Can you work these out from the drawing? Everything is in mm from the part's minimum corner. A direction names the side the tool comes from. Give positions to 0.01 mm unless a question says otherwise; leave off trailing zeros. One line per question, with ' | ' between items.
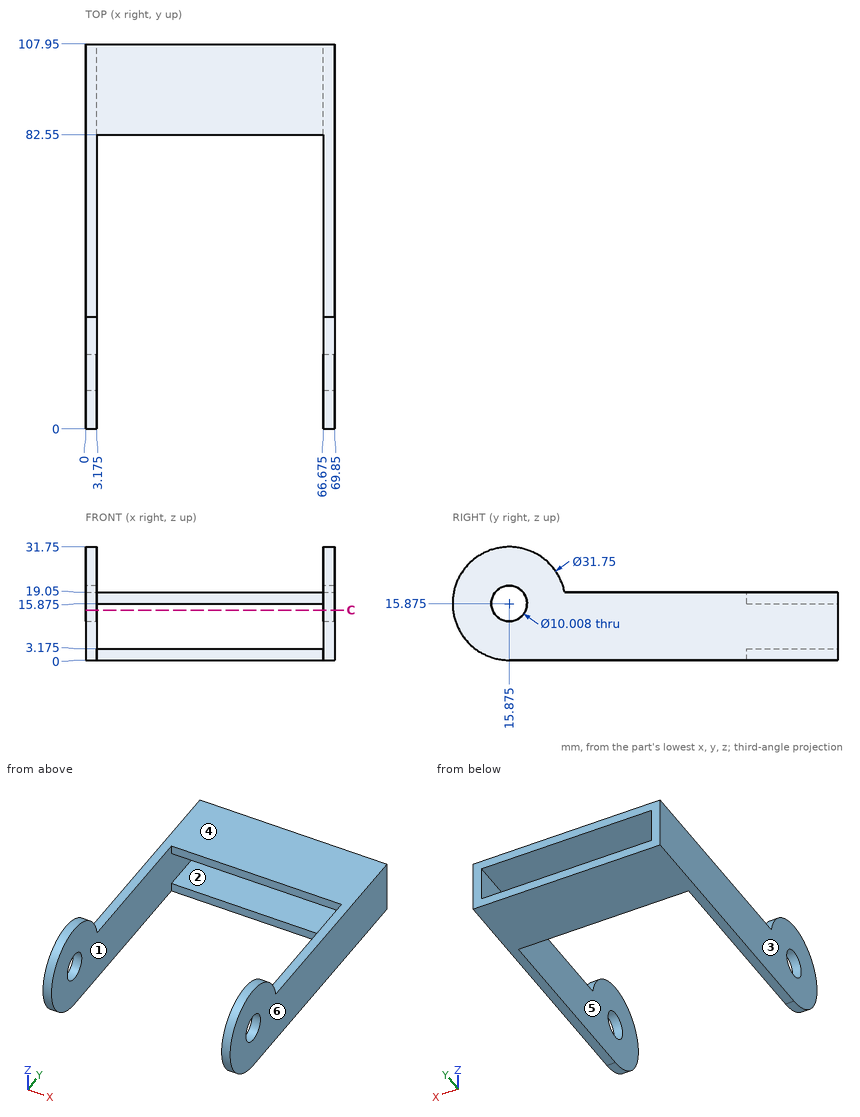
1) Thinking about a two-plate mould opening in X: for the marked faces 4, 5 and 6, which applies, +X half, -X half, draft (parallel to the pull), parting line (faces both ways), or undercut?
Model answer:
face 4: draft | face 5: undercut | face 6: +X half
2) On a 3-axis mill with a long thin cutter (end or side, diameter ignored), from which of +Z, -Z, +X, -X, +Y, -Y can I reach the whole of each face in a straight line? I mean the marked faces 1, 2 and 3. Say none if no direction works.
Model answer:
face 1: -Y | face 2: +Y, -Y | face 3: +Z, -Z, -X, +Y, -Y
3) I want a section at C-C (z = 14). State how many separate pieces and enclosed holes the cut face has, plus the area to 3 significant figures.
Model answer:
separate pieces: 4 | enclosed holes: 0 | area: 626 mm2
4) Please list where this line runs through material, in increasing order: L1, parallel to Y at x = 5, z = 16.5.
Model answer:
L1: y = 82.55 to 107.95
5) I'm going to push flat-ended pins straight in: P1, Ø3.5, axis at x = 48, z = 1, coming from the -Y side; P2, Ø6, axis at x = 11.5, y = 90, coming from the +Z side. Where does each tip first touch, or does it pass through?
Model answer:
P1: stops at y = 82.55 | P2: stops at z = 19.05
